The model under review builds one solid part; all positions refer to its coordinate system, in mm. Give positions to 0.01 mm unless a question says otherwise; leave off trailing zeros. Order: outer loops, then holes, each group sorted by start corner. A loop starts at its lowest first (then second) coordinate and runs counter-clockwise, first axis right, second up. Notation, with made-up numbers: (-29, -8) - (-8, -8) arc R23 cw to (-8, 27) - close; hole circle Ø5 at (12.25, -38.75). An arc over 180 degrees is marked (long way). Answer as CSV lines item,"result". Start each with the question number.
from build123d import *

# Parameters (mm, degrees)
F1_DEPTH  = 505
F2_W      = 10
F2_H      = 10
F3_DEPTH  = 1
F4_W      = 505
F4_H      = 10
F5_DEPTH  = 505
F7_DEPTH  = 10.001
F8_DEPTH  = 10.001
F10_DEPTH = 10.001
F11_R     = 10


with BuildPart() as f1:
    # F0 (on Right) → F1 (new body)
    with BuildSketch(Plane.YZ):
        Polygon((-1, 2), (-1, 0), (-1, -2), (-5, -2), (-5, -5), (0, -5), (5, -5), (5, -2), (1, -2), (1, 0), (1, 2), (5, 2), (5, 5), (0, 5), (-5, 5), (-5, 2), align=None)
    extrude(amount=F1_DEPTH)

    # F2 (on face) → F3 (join)
    with BuildSketch(Plane.XY.offset(5)):
        with Locations((500, 0)):
            Rectangle(F2_W, F2_H)
    extrude(amount=F3_DEPTH)

    # F4 (on face) → F5 (join)
    with BuildSketch(Plane(origin=(0, 0, -5), x_dir=(1, 0, 0), z_dir=(0, 0, -1))):
        with Locations((252.5, 0)):
            Rectangle(F4_W, F4_H)
    extrude(amount=F5_DEPTH)

    # F6 (on face) → F7 (cut, through all)
    with BuildSketch(Plane.XZ.offset(5)):
        Polygon((0, -5), (0, -463), (458, -5), align=None)
    extrude(amount=-F7_DEPTH, mode=Mode.SUBTRACT)

    # F6 (on face) → F8 (cut, through all)
    with BuildSketch(Plane.XZ.offset(5)):
        Polygon((0, -5), (0, -463), (458, -5), align=None)
    extrude(amount=-F8_DEPTH, mode=Mode.SUBTRACT)

    # F9 (on face) → F10 (cut, through all)
    with BuildSketch(Plane.XZ.offset(5)):
        Polygon((505, -5), (0, -510), (505, -510), align=None)
    extrude(amount=-F10_DEPTH, mode=Mode.SUBTRACT)

    # F11
    f11_edges = [f1.edges().sort_by_distance(p)[0] for p in [
        (458, 0, -5),
    ]]
    fillet(f11_edges, radius=F11_R)


solid = f1.part
Item 1: Take a section at B-B on x = 42. Write out the cut boundary in (y, z).
Item 2: Mouldability with a two-part tool opening along Z and no side actions: class faces 1 (the face through (217, 0, -246)), 2 (the face through (256, 0, -254)), 3 (the face through (251, 5, -255)) as released by +Z, released by -Z, zero draft, split by the parting line, or undercut.
Item 3: Clearance check with flat-ended pins moving along their axes: pin 1 (1 mm diameter, centred on x = 119.5, y = -1, fed in from -Z); pin 2 (3 mm diameter, centred on x = 203.5, y = 3, fed in from +Z); pin 3 (1.2 mm diameter, centred on x = 324, y = 3.5, fed in from -Z); pin 4 (4.5 mm diameter, centred on x = 204.5, z = 0, fed in from +Y). State where each tip first meets the part, or that it passes through.
Item 4: Take a section at A-A on y = 2.5. Write out the cut boundary in (x, z), and give its area (3 significant figures).
Item 5: Take a section at C-C on z = -40. Write out the cut boundary in (x, y).
Item 6: For line 1 along Z through (x, y) = (174.5, 2); line 2 along Z through (x, y) = (359, -2.25); line 3 along Z through (x, y) = (481, -3.25), list the stretches that pass through material, from the lowest coordinate up.
Data:
1,outline,"(-5, -468) - (5, -468) - (5, -421) - (-5, -421) - close; (-5, -5) - (5, -5) - (5, -2) - (1, -2) - (1, 2) - (5, 2) - (5, 5) - (-5, 5) - (-5, 2) - (-1, 2) - (-1, -2) - (-5, -2) - close"
2,face 1,"undercut"
2,face 2,"released by -Z"
2,face 3,"zero draft"
3,pin 1,"stops at z = -391"
3,pin 2,"stops at z = 5"
3,pin 3,"stops at z = -186.6"
3,pin 4,"stops at y = 5"
4,outline,"(0, -510) - (505, -5) - (505, -2) - (0, -2) - (0, -5) - (433.86, -5) arc R10 cw to (440.93, -22.07) - (0, -463) - close; (0, 2) - (505, 2) - (505, 6) - (495, 6) - (495, 5) - (0, 5) - close"
4,area,"25,800 mm^2"
5,outline,"(423, -5) - (470, -5) - (470, 5) - (423, 5) - close"
6,line 1,"z = -335.5 to -288.5, -5 to -2, 2 to 5"
6,line 2,"z = -151 to -104, -5 to -2, 2 to 5"
6,line 3,"z = -29 to -2, 2 to 5"
